```python
from build123d import *

# Parameters (mm, degrees)
SKETCH1_R           = 3.429
SKETCH1_R_2         = 2.54
BOSS_EXTRUDE1_DEPTH = 3.2004
SKETCH2_R           = 1.7272
CUT_EXTRUDE1_DEPTH  = 3.2004
SKETCH5_R           = 1.7272
SKETCH5_W           = 40.894
SKETCH5_H           = 20.32
CUT_EXTRUDE3_DEPTH  = 4.2004
CUT_EXTRUDE4_DEPTH  = 3.2004
SKETCH9_R           = 13.885201093
CUT_EXTRUDE7_DEPTH  = 3.2004
SKETCH10_R          = 3.429
BOSS_EXTRUDE2_DEPTH = 3.2004
FILLET1_R           = 6.35


with BuildPart() as part:
    # Sketch1 → Boss-Extrude1 (new body)
    with BuildSketch(Plane.XY):
        with BuildLine():
            Line((0, 0), (120.015, 0))
            ThreePointArc((120.015, 0), (130.351788397, 3.075697789), (137.325636158, 11.302152593))
            Line((137.325636158, 11.302152593), (149.69326877, 39.451329485))
            ThreePointArc((149.69326877, 39.451329485), (148.774539583, 50.600046625), (138.937102863, 55.925719911))
            Line((138.937102863, 55.925719911), (-26.54325766, 55.925719911))
            ThreePointArc((-26.54325766, 55.925719911), (-36.046025914, 50.429200208), (-36.019801229, 39.451329485))
            Line((-36.019801229, 39.451329485), (-19.648099871, 11.302152593))
            ThreePointArc((-19.648099871, 11.302152593), (-11.333429333, 3.027112684), (0, 0))
        make_face()
        with Locations((120.015, 18.90776)):
            Circle(SKETCH1_R, mode=Mode.SUBTRACT)
        with Locations((0, 18.90776)):
            Circle(SKETCH1_R, mode=Mode.SUBTRACT)
        with Locations((19.734727626, 25.566426992)):
            Circle(SKETCH1_R_2, mode=Mode.SUBTRACT)
    extrude(amount=BOSS_EXTRUDE1_DEPTH)

    # Sketch2 → Cut-Extrude1 (cut)
    with BuildSketch(Plane(origin=(0, 0, 0), x_dir=(-1, 0, 0), z_dir=(0, 0, -1))):
        with Locations((-92.0115, 52.115719911)):
            Circle(SKETCH2_R)
        with Locations((-28.0035, 52.115719911)):
            Circle(SKETCH2_R)
        with Locations((-98.1075, 3.81)):
            Circle(SKETCH2_R)
        with Locations((-21.9075, 3.81)):
            Circle(SKETCH2_R)
    extrude(amount=-CUT_EXTRUDE1_DEPTH, mode=Mode.SUBTRACT)

    # Sketch5 → Cut-Extrude3 (cut, through all)
    with BuildSketch(Plane(origin=(0, 0, 0), x_dir=(-1, 0, 0), z_dir=(0, 0, -1))):
        with Locations((-79.746999972, 23.90776)):
            Circle(SKETCH5_R)
        with Locations((-29.246999972, 13.90776)):
            Circle(SKETCH5_R)
        with Locations((-29.246999972, 23.90776)):
            Circle(SKETCH5_R)
        with Locations((-79.746999972, 13.90776)):
            Circle(SKETCH5_R)
        with Locations((-54.496999972, 18.90776)):
            Rectangle(SKETCH5_W, SKETCH5_H)
    extrude(amount=-CUT_EXTRUDE3_DEPTH, mode=Mode.SUBTRACT)

    # Sketch6 → Cut-Extrude4 (cut)
    with BuildSketch(Plane.XY.offset(3.2004)):
        with BuildLine():
            Line((29.985999972, 19.92376), (34.049999972, 19.92376))
            Line((34.049999972, 19.92376), (34.049999972, 17.89176))
            Line((34.049999972, 17.89176), (29.985999972, 17.89176))
            ThreePointArc((29.985999972, 17.89176), (28.969999972, 18.90776), (29.985999972, 19.92376))
        make_face()
        with BuildLine():
            Line((74.943999972, 19.92376), (79.007999972, 19.92376))
            ThreePointArc((79.007999972, 19.92376), (80.023999972, 18.90776), (79.007999972, 17.89176))
            Line((79.007999972, 17.89176), (74.943999972, 17.89176))
            Line((74.943999972, 17.89176), (74.943999972, 19.92376))
        make_face()
    extrude(amount=-CUT_EXTRUDE4_DEPTH, mode=Mode.SUBTRACT)

    # Sketch9 → Cut-Extrude7 (cut)
    with BuildSketch(Plane(origin=(0, 0, 0), x_dir=(-1, 0, 0), z_dir=(0, 0, -1))):
        with Locations((-49.53, 18.90776)):
            Circle(SKETCH9_R)
    extrude(amount=-CUT_EXTRUDE7_DEPTH, mode=Mode.SUBTRACT)

    # Sketch10 → Boss-Extrude2 (add)
    with BuildSketch(Plane.XY.offset(3.2004)):
        Polygon((72.5805, 80.055719911), (110.6805, 80.055719911), (117.0305, 55.925719911), (66.2305, 55.925719911), align=None)
        with Locations((78.9305, 67.990719911)):
            Circle(SKETCH10_R, mode=Mode.SUBTRACT)
        with Locations((104.3305, 67.990719911)):
            Circle(SKETCH10_R, mode=Mode.SUBTRACT)
    extrude(amount=-BOSS_EXTRUDE2_DEPTH)

    # Fillet1
    fillet1_edges = [part.edges().sort_by_distance(p)[0] for p in [
        (117.0305, 55.925719911, 1.6002),
        (110.6805, 80.055719911, 1.6002),
        (72.5805, 80.055719911, 1.6002),
        (66.2305, 55.925719911, 1.6002),
    ]]
    fillet(fillet1_edges, radius=FILLET1_R)


solid = part.part
```
Check sheet for the modelled part. Datum: model origin and axes. Units: mm. A direction names the side the tool comes from. Give positions to 0.01 mm unless a question says otherwise; leave off trailing zeros. Loops run counter-clockwise (first coordinate to the right, second up) from the corner with the lowest first, then second, coordinate; pieces in that order, holes last. Notation, with made-up numbers: M 28.5,-34 L 79.5,-34 A19 cw 79.5,-3 Z; hole C 18,-17.75 d4. An arc over 180 degrees is marked long. Answer in a Markdown table with one row per item.
1) Thickness scan on line 1 (Y direction, x = 39, z = 1.3); line 2 (Y direction, x = 30.5, z = 0.6); line 3 (Y direction, x = 29.5, z = 0.35). Record the ranges inside material, lowest first.
Solutions:
| item | result |
|---|---|
| line 1 | y = 0 to 8.75, 29.07 to 55.93 |
| line 2 | y = 0 to 12.72, 15.1 to 17.89, 19.92 to 22.72, 25.1 to 55.93 |
| line 3 | y = 0 to 12.2, 15.62 to 18.02, 19.8 to 22.2, 25.62 to 51.25, 52.98 to 55.93 |
2) Mould release check, pull along X, two halves, no side actions. Record for faces 3 (the face through (109.71, 78.7, 1.58)), 4 (the face through (-27.949, 25.574, 1.578)), 5 (the face through (93.285, 53.283, 1.578)): released by +X, released by -X, zero draft, split by the parting line, or undercut.
Solutions:
| item | result |
|---|---|
| face 3 | released by +X |
| face 4 | released by -X |
| face 5 | undercut |
3) Cross-section at A-A (x = 63). Enter the section's corners in (y, z), plus the area to 3 significant figures.
Solutions:
| item | result |
|---|---|
| outline | M 0,0 L 8.75,0 L 8.75,3.2 L 0,3.2 Z; M 29.07,0 L 56.15,0 L 56.15,3.2 L 29.07,3.2 Z |
| area | 115 mm^2 |
4) Cross-section at B-B (z = 0.65). Count the separate pieces of the cut face and the enclosed holes in it, plus the area to 3 significant figures.
Solutions:
| item | result |
|---|---|
| separate pieces | 1 |
| enclosed holes | 14 |
| area | 9,400 mm^2 |
5) Tool access check on faces 1 (the face through (91, 80.056, 2)), 2 (the face through (74.944, 13, 2)). Record the directions out of +Z, -Z, +X, -X, +Y, -Y that give a thin tool (end or side, any length) a straight path to the whole face; none if there is none.
Solutions:
| item | result |
|---|---|
| face 1 | +Z, -Z, +X, -X, +Y |
| face 2 | +Z, -Z |
6) Cross-section at D-D (y = 35). Enter the section's corners in (x, z).
Solutions:
| item | result |
|---|---|
| outline | M -33.43,0 L 147.74,0 L 147.74,3.2 L -33.43,3.2 Z |
7) Cross-section at C-C (x = 127.5). Enter the section's corners in (y, z).
Solutions:
| item | result |
|---|---|
| outline | M 1.54,0 L 55.93,0 L 55.93,3.2 L 1.54,3.2 Z |
